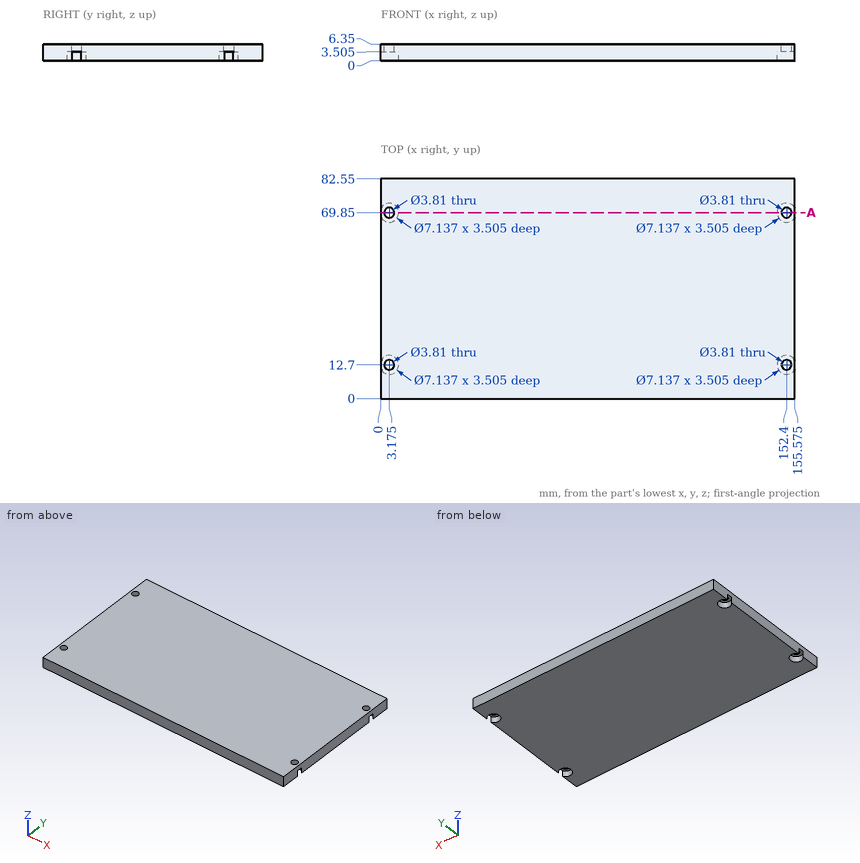
Geometry check sheet. Reference: drawing and pictorial views, mm from the part's lowest x, y, z. Give positions to 0.01 mm unless a question says otherwise; leave off trailing zeros. Use CSV: the item, a comma, the result in double quotes. Start each with the question number.
1) Sectioned sample at A-A, the plane y = 69.85. Give the number of separate pieces and of enclosed holes in the cut face, plus the area to 3 significant figures.
2) Material ranges on line 1 (X direction, y = 12.7, z = 4.5) (1 decimal); line 2 (Y direction, x = 152.4, z = 0.8), recorded low to high. Write a range as from..to.
3) Go/stop test with a flat-tipped pin: P1, Ø2, axis at x = 153.5, y = 70.5, coming from the -Z side (1 decimal). Record where the tip stops, or that it passes through.
Recorded:
1,separate pieces,"3"
1,enclosed holes,"0"
1,area,"919 mm2"
2,line 1,"0..1.3, 5.1..150.5, 154.3..155.6"
2,line 2,"0..9.13, 16.27..66.28, 73.42..82.55"
3,P1,"z = 3.5"
